Design review of the part built by this model. Coordinates are the model's own, in mm. Round coordinates to 2 decimals unless told otherwise and drop trailing zeros. Order: outer loops, then holes, each group sorted by start corner. A loop starts at its lowest first (then second) coordinate and runs counter-clockwise, first axis right, second up. Notation, with made-up numbers: M 86.25,20 L 105.25,20 A36 ccw 105.25,57 Z; hole C 16,-18.75 d2. An arc over 180 degrees is marked long. Use a Markdown table: item, result. Add a question column.
(1) Take a section at B-B (z = -1.75). Count the separate pieces of the cut face and the enclosed holes in it, then the cut area to 3 significant figures.
(2) Take a section at C-C (y = 1.75). Write out the cut boundary in (x, z).
(3) Take a section at A-A (x = 9.25). Write out the cut boundary in (y, z).
(4) For pin 1 (0.6 mm diameter, centred on y = 1, z = -1, fed in from +X); pin 2 (0.9 mm diameter, centred on x = 4, z = -1, fed in from +Y), all flat-tipped, find the tip position at first contact; note any pin that passes through.
(5) To check wall thickness, follow probe 1 along Y at (x, z) = (14.25, 7); probe 2 along Y at (x, z) = (16.5, -1.5); probe 3 along Z at (x, y) = (2, 4.35). State the ranges of each line that lie inside material, in increasing order. Write a range as from..to.
```python
from build123d import *

# Parameters (mm, degrees)
SKICA1_W                 = 18.2
SKICA1_H                 = 5
P_IDAT_VYSUNUT_M1_DEPTH  = 8.4
SKICA3_W                 = 0.8
SKICA3_H                 = 0.8
ODEBRAT_VYSUNUT_M1_DEPTH = 6
SKICA6_W                 = 0.8
SKICA6_H                 = 0.8
P_IDAT_VYSUNUT_M2_DEPTH  = 2.8


with BuildPart() as part:
    # Skica1 → Přidat vysunutím1 (new body)
    with BuildSketch(Plane.XY):
        with Locations((9.1, 2.5)):
            Rectangle(SKICA1_W, SKICA1_H)
    extrude(amount=P_IDAT_VYSUNUT_M1_DEPTH)

    # Skica3 → Odebrat vysunutím1 (cut)
    with BuildSketch(Plane.XY.offset(8.4)):
        with Locations((1.45, 3.682710822)):
            Rectangle(SKICA3_W, SKICA3_H)
        with Locations((1.45, 1.082710822)):
            Rectangle(SKICA3_W, SKICA3_H)
        with Locations((6.55, 3.682710822)):
            Rectangle(SKICA3_W, SKICA3_H)
        with Locations((4, 3.682710822)):
            Rectangle(SKICA3_W, SKICA3_H)
        with Locations((4, 1.082710822)):
            Rectangle(SKICA3_W, SKICA3_H)
        with Locations((6.55, 1.082710822)):
            Rectangle(SKICA3_W, SKICA3_H)
        with Locations((9.1, 3.682710822)):
            Rectangle(SKICA3_W, SKICA3_H)
        with Locations((9.1, 1.082710822)):
            Rectangle(SKICA3_W, SKICA3_H)
        with Locations((11.65, 3.682710822)):
            Rectangle(SKICA3_W, SKICA3_H)
        with Locations((11.65, 1.082710822)):
            Rectangle(SKICA3_W, SKICA3_H)
        with Locations((14.2, 3.682710822)):
            Rectangle(SKICA3_W, SKICA3_H)
        with Locations((14.2, 1.082710822)):
            Rectangle(SKICA3_W, SKICA3_H)
        with Locations((16.75, 3.682710822)):
            Rectangle(SKICA3_W, SKICA3_H)
        with Locations((16.75, 1.082710822)):
            Rectangle(SKICA3_W, SKICA3_H)
    extrude(amount=-ODEBRAT_VYSUNUT_M1_DEPTH, mode=Mode.SUBTRACT)

    # Skica6 → Přidat vysunutím2 (add)
    with BuildSketch(Plane(origin=(0, 0, 0), x_dir=(-1, 0, 0), z_dir=(0, 0, -1))):
        with Locations((-1.45, 3.682710822)):
            Rectangle(SKICA6_W, SKICA6_H)
        with Locations((-4, 3.682710822)):
            Rectangle(SKICA6_W, SKICA6_H)
        with Locations((-6.55, 3.682710822)):
            Rectangle(SKICA6_W, SKICA6_H)
        with Locations((-9.1, 3.682710822)):
            Rectangle(SKICA6_W, SKICA6_H)
        with Locations((-11.65, 3.682710822)):
            Rectangle(SKICA6_W, SKICA6_H)
        with Locations((-14.2, 3.682710822)):
            Rectangle(SKICA6_W, SKICA6_H)
        with Locations((-16.75, 3.682710822)):
            Rectangle(SKICA6_W, SKICA6_H)
        with Locations((-1.45, 1.082710822)):
            Rectangle(SKICA6_W, SKICA6_H)
        with Locations((-4, 1.082710822)):
            Rectangle(SKICA6_W, SKICA6_H)
        with Locations((-6.55, 1.082710822)):
            Rectangle(SKICA6_W, SKICA6_H)
        with Locations((-9.1, 1.082710822)):
            Rectangle(SKICA6_W, SKICA6_H)
        with Locations((-11.65, 1.082710822)):
            Rectangle(SKICA6_W, SKICA6_H)
        with Locations((-14.2, 1.082710822)):
            Rectangle(SKICA6_W, SKICA6_H)
        with Locations((-16.75, 1.082710822)):
            Rectangle(SKICA6_W, SKICA6_H)
    extrude(amount=P_IDAT_VYSUNUT_M2_DEPTH)


solid = part.part
```
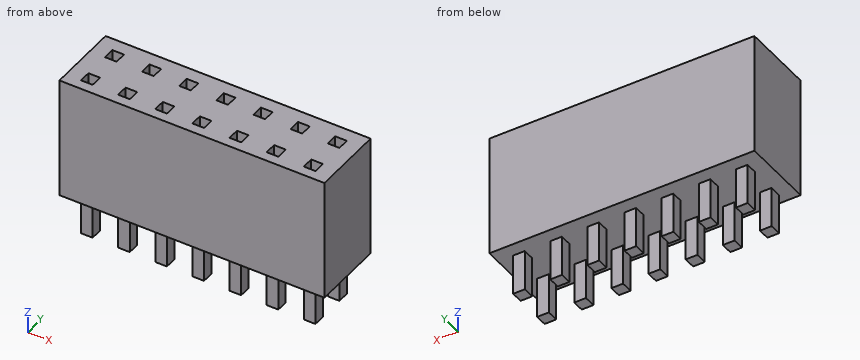
Verdict:
| question | item | result |
|---|---|---|
| 1 | separate pieces | 14 |
| 1 | enclosed holes | 0 |
| 1 | area | 8.96 mm^2 |
| 2 | outline | M 0,0 L 18.2,0 L 18.2,8.4 L 0,8.4 Z |
| 3 | outline | M 0,0 L 0.68,0 L 0.68,-2.8 L 1.48,-2.8 L 1.48,0 L 3.28,0 L 3.28,-2.8 L 4.08,-2.8 L 4.08,0 L 5,0 L 5,8.4 L 4.08,8.4 L 4.08,2.4 L 3.28,2.4 L 3.28,8.4 L 1.48,8.4 L 1.48,2.4 L 0.68,2.4 L 0.68,8.4 L 0,8.4 Z |
| 4 | pin 1 | stops at x = 17.15 |
| 4 | pin 2 | stops at y = 4.08 |
| 5 | probe 1 | y = 0..0.68, 1.48..3.28, 4.08..5 |
| 5 | probe 2 | y = 0.68..1.48, 3.28..4.08 |
| 5 | probe 3 | z = 0..8.4 |
